Part model, mm, in its own coordinate system. A direction names the side the tool comes from. Coordinates: 2 decimals unless noted, no trailing zeros. Use a Markdown table: item, result. Add a question column.
1. Pull direction Z, two halves, no side cores. Call faces 4 (the flat face through (-56.6, 2.515, -32.2)), 5 (the cylindrical face through (13.77, 11.39, -61.99)), 6 (the flat face through (-46.5, 6.542, -37.7)): pulls with the +Z half, pulls with the -Z half, needs draft (parallel to the pull), parting line crosses it, or undercut.
2. Drop flat-ended pins along their axis: pin 1 (3.5 mm diameter, centred on x = 57.74, z = 33.34, fed in from +Y) (3 decimals); pin 2 (3.5 mm diameter, centred on x = -57.74, z = -33.34, fed in from -Y); pin 3 (3 mm diameter, centred on x = 1, y = 6.5, fed in from +Z). Give the stop position or say it passes through.
3. Wall check: probe 1 along Y at (x, z) = (-61.5, 8.5); probe 2 along Z at (x, y) = (1, 7.75); probe 3 along Y at (x, z) = (-14, -10.5). Give the ranges that are in metal, low to high. Write a range as [from, to].
4. 3-axis set-ups, long thin cutter, end or side, ignore diameter. For faces 1 (the flat face through (-46.5, 4.179, -37.7)), 2 (the cylindrical face through (13.77, 7.29, -61.99)), 3 (the cylindrical face through (59.486, 1.24, 35.239)): which of +Z, -Z, +X, -X, +Y, -Y reach the whole face in a straight line?
from build123d import *

# Parameters (mm, degrees)
SKETCH1_R                                      = 79.248
EXTRUDE1_DEPTH                                 = 3.175
SKETCH2_R                                      = 63.5
EXTRUDE2_DEPTH                                 = 9.2075
SKETCH4_W                                      = 3.81
SKETCH4_H                                      = 2.3622
CHAMFER1_SIZE                                  = 0.381
SKETCH8_R                                      = 57.15
CUT_EXTRUDE1_DEPTH                             = 8.89
CBORE_FOR_3_SOCKET_HEAD_CAP_SCREW1_D           = 2.794
CBORE_FOR_3_SOCKET_HEAD_CAP_SCREW1_CBORE_D     = 5.15874
CBORE_FOR_3_SOCKET_HEAD_CAP_SCREW1_CBORE_DEPTH = 2.5146
CIRPATTERN1_COUNT                              = 6


with BuildPart() as part:
    # Sketch1 → Extrude1 (new body)
    with BuildSketch(Plane(origin=(0, 0, 0), x_dir=(1, 0, 0), z_dir=(0, 1, 0))):
        Circle(SKETCH1_R)
    extrude(amount=EXTRUDE1_DEPTH)

    # Sketch2 → Extrude2 (add)
    with BuildSketch(Plane(origin=(0, 3.175, 0), x_dir=(-1, 0, 0), z_dir=(0, 1, 0))):
        Circle(SKETCH2_R)
    extrude(amount=EXTRUDE2_DEPTH)

    # Sketch4 → Cut-Revolve7 (revolve, cut)
    with BuildSketch(Plane(origin=(0, 0, 0), x_dir=(0, 0, -1), z_dir=(1, 0, 0))):
        with Locations((-61.595, 9.224034757)):
            Rectangle(SKETCH4_W, SKETCH4_H)
        with Locations((-61.595, 5.360539726)):
            Rectangle(SKETCH4_W, SKETCH4_H)
    revolve(axis=Axis((0, 0, 0), (0, 1, 0)), mode=Mode.SUBTRACT)

    # Chamfer1
    chamfer1_edges = [part.edges().sort_by_distance(p)[0] for p in [
        (63.5, 10.405134757, 0),
        (63.5, 8.042934757, 0),
        (63.5, 6.541639726, 0),
        (63.5, 4.179439726, 0),
        (63.5, 12.3825, 0),
    ]]
    chamfer(chamfer1_edges, length=CHAMFER1_SIZE)

    # Sketch8 → Cut-Extrude1 (cut)
    with BuildSketch(Plane(origin=(0, 12.3825, 0), x_dir=(1, 0, 0), z_dir=(0, 1, 0))):
        Circle(SKETCH8_R)
    extrude(amount=-CUT_EXTRUDE1_DEPTH, mode=Mode.SUBTRACT)

    # CBORE for _3 Socket Head Cap Screw1 (through all)
    with Locations(Plane(origin=(57.742243797, 0, 33.3375), x_dir=(0, 0, -1), z_dir=(0, -1, 0))):
        with Locations((0, 0)):
            cbore_for_3_socket_head_cap_screw1 = CounterBoreHole(CBORE_FOR_3_SOCKET_HEAD_CAP_SCREW1_D / 2, CBORE_FOR_3_SOCKET_HEAD_CAP_SCREW1_CBORE_D / 2, CBORE_FOR_3_SOCKET_HEAD_CAP_SCREW1_CBORE_DEPTH)

    # CirPattern1: CBORE for _3 Socket Head Cap Screw1 ×6 about axis
    cirpattern1_axis = Axis((0, 0, 0), (0, 1, 0))
    for i in range(1, CIRPATTERN1_COUNT):
        add(cbore_for_3_socket_head_cap_screw1.rotate(cirpattern1_axis, i * 360 / CIRPATTERN1_COUNT), mode=Mode.SUBTRACT)


solid = part.part
Geometry check:
| question | item | result |
|---|---|---|
| 1 | face 4 | undercut |
| 1 | face 5 | parting line crosses it |
| 1 | face 6 | needs draft |
| 2 | pin 1 | stops at y = 3.175 |
| 2 | pin 2 | stops at y = 2.51 |
| 2 | pin 3 | stops at z = 63.5 |
| 3 | probe 1 | y = [0, 4.18], [6.54, 8.04], [10.41, 12.38] |
| 3 | probe 2 | z = [-63.4, -57.14], [57.14, 63.4] |
| 3 | probe 3 | y = [0, 3.49] |
| 4 | face 1 | none |
| 4 | face 2 | +Y |
| 4 | face 3 | -Y |
